```python
from build123d import *

# Parameters (mm, degrees)
F0_W     = 65.872892
F0_H     = 35.192366
F1_DEPTH = 25.4
F2_T     = -0.1
F3_R     = 7.692897
F4_DEPTH = 42.926


with BuildPart() as f1:
    # F0 (on Front) → F1 (new body)
    with BuildSketch(Plane.XZ):
        Rectangle(F0_W, F0_H)
    extrude(amount=F1_DEPTH)

    # F2
    f2_openings = [f1.faces().sort_by_distance(p)[0] for p in [
        (0, -12.7, -17.596183),
    ]]
    offset(amount=F2_T, openings=f2_openings)

    # F3 (on face) → F4 (cut)
    with BuildSketch(Plane.XZ.offset(25.4)):
        with Locations((-3.789655, 0)):
            Circle(F3_R)
    extrude(amount=-F4_DEPTH, mode=Mode.SUBTRACT)


solid = f1.part
```
Design review of the part built by this model. Coordinates are the model's own, in mm. Give positions to 0.01 mm unless a question says otherwise; leave off trailing zeros. Write each loop counter-clockwise with the first axis right and the second up, starting at its lowest first coordinate (ties: lowest second). Pieces come first, ordered by that corner, then holes. Notation, with made-up numbers: (85, 60) - (125, 60) arc R26 ccw to (125, 92) - close; hole circle Ø6 at (81, 31). An arc over 180 degrees is marked (long way). Return JSON: item names as keys, results as strings. Group by question number.
(1) We need section C-C, the plane y = -12.5. Give the boundary of the cut face in (x, z), then the cut area to 3 significant figures.
(2) We need section A-A, the plane x = -10.5. Give the boundary of the cut face in (y, z).
(3) Insertion check: pin 1 (1.5 mm diameter, centred on x = -9, y = -14, fed in from -Z). The pin has a flat end and moves straight along its axis. Give the tip position at first contact, or say it passes through.
(4) We need section B-B, the plane z = 0. Give the boundary of the cut face in (x, y), then the cut area to 3 significant figures.
(5) We need section D-D, the plane x = -21. Give the boundary of the cut face in (y, z), then the cut area to 3 significant figures.
Reported:
{
 "1": {"outline": "(-32.94, -17.6) - (-32.84, -17.6) - (-32.84, 17.5) - (32.84, 17.5) - (32.84, -17.6) - (32.94, -17.6) - (32.94, 17.6) - (-32.94, 17.6) - close", "area": "13.6 mm2"},
 "2": {"outline": "(-25.4, -17.6) - (-25.3, -17.6) - (-25.3, -3.76) - (-25.4, -3.76) - close; (-25.4, 3.76) - (-25.3, 3.76) - (-25.3, 17.5) - (-0.1, 17.5) - (-0.1, 3.76) - (0, 3.76) - (0, 17.6) - (-25.4, 17.6) - close; (-0.1, -17.6) - (0, -17.6) - (0, -3.76) - (-0.1, -3.76) - close"},
 "3": {"pin 1": "stops at z = 17.5"},
 "4": {"outline": "(-32.94, -25.4) - (-11.48, -25.4) - (-11.48, -25.3) - (-32.84, -25.3) - (-32.84, -0.1) - (-11.48, -0.1) - (-11.48, 0) - (-32.94, 0) - close; (3.9, -25.4) - (32.94, -25.4) - (32.94, 0) - (3.9, 0) - (3.9, -0.1) - (32.84, -0.1) - (32.84, -25.3) - (3.9, -25.3) - close", "area": "15.1 mm2"},
 "5": {"outline": "(-25.4, -17.6) - (-25.3, -17.6) - (-25.3, 17.5) - (-0.1, 17.5) - (-0.1, -17.6) - (0, -17.6) - (0, 17.6) - (-25.4, 17.6) - close", "area": "9.56 mm2"}
}
